Source: CAD feature listing. Evaluate the final solid. Frame: model axes, mm. Give positions to 0.01 mm unless a question says otherwise; leave off trailing zeros. Write each loop counter-clockwise with the first axis right and the second up, starting at its lowest first coordinate (ties: lowest second). Pieces come first, ordered by that corner, then holes. Notation, with made-up numbers: M -10.75,19 L -2.75,19 A22 cw -2.75,40 Z; hole C 44,39.25 d2. An arc over 180 degrees is marked long. Answer as a JSON object with one key per item and string values. Group by question number.
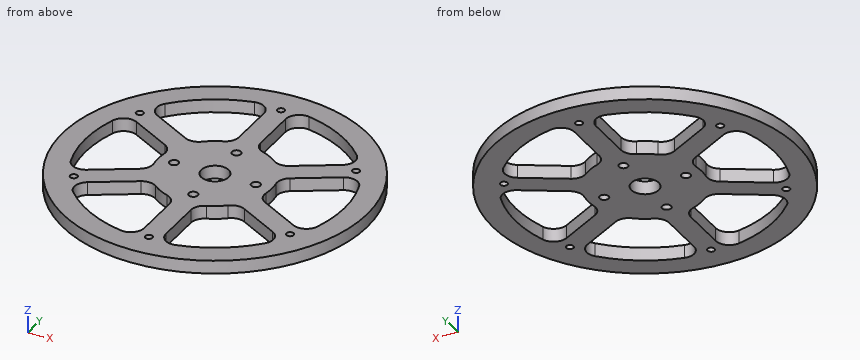
Autodesk Inventor part; units mm, degrees
ref_plane "YZ Plane" through (0, 0, 0) normal (1, 0, 0) x (0, 1, 0)
ref_plane "XZ Plane" through (0, 0, 0) normal (0, 1, 0) x (-1, 0, 0)
ref_plane "XY Plane" through (0, 0, 0) normal (0, 0, 1) x (1, 0, 0)
sketch "スケッチ1" plane through (0, 0, 0) normal (0, 0, 1) x (1, 0, 0)
  circle A0 centre (0, 0) radius 67
  circle A1 centre (0, 0) radius 57
  circle A2 centre (0, 0) radius 25
  line L0 (0, 0) -> (0, 67)
  circle A3 centre (0, 0) radius 6.05
  line L1 (4.7669, 0.7625) -> (4.7669, 66.8302)
  line L2 (4.7669, 0.7625) -> (70.8346, 0.7625) construction
  line L3 (-4.7669, 0.7625) -> (-4.7669, 66.8302)
  line L4 (-3.0438, -3.747) -> (-60.2601, 29.2869)
  line L5 (1.7231, 4.5095) -> (-55.4932, 37.5433)
  line L6 (1.7231, -4.5095) -> (-55.4932, -37.5433)
  line L7 (-3.0438, 3.747) -> (-60.2601, -29.2869)
  line L8 (4.7669, -0.7625) -> (4.7669, -66.8302)
  line L9 (-4.7669, -0.7625) -> (-4.7669, -66.8302)
  line L10 (3.0438, 3.747) -> (60.2601, -29.2869)
  line L11 (-1.7231, -4.5095) -> (55.4932, -37.5433)
  line L12 (-1.7231, 4.5095) -> (55.4932, 37.5433)
  line L13 (3.0438, -3.747) -> (60.2601, 29.2869)
  point P0 (4.7669, 56.8003)
  point P1 (46.8071, 32.5284)
  point P2 (18.87, 16.3989)
  point P3 (4.7669, 24.5413)
  point P4 (-4.7669, 56.8003)
  point P5 (-4.7669, 24.5413)
  point P6 (-18.87, 16.3989)
  point P7 (-46.8071, 32.5284)
  point P8 (51.574, -24.2719)
  point P9 (23.6368, -8.1424)
  point P10 (23.6368, 8.1424)
  point P11 (51.574, 24.2719)
  point P12 (4.7669, -56.8003)
  point P13 (4.7669, -24.5413)
  point P14 (18.87, -16.3989)
  point P15 (46.8071, -32.5284)
  point P16 (-46.8071, -32.5284)
  point P17 (-18.87, -16.3989)
  point P18 (-4.7669, -24.5413)
  point P19 (-4.7669, -56.8003)
  point P20 (-51.574, 24.2719)
  point P21 (-23.6368, 8.1424)
  point P22 (-23.6368, -8.1424)
  point P23 (-51.574, -24.2719)
  dimension "d0" = 134
  dimension "d1" = 114
  dimension "d2" = 50
  dimension "d3" = 12.1
  dimension "d4" = 90
  dimension "d7" = 360
extrude "押し出し1" add sketch "スケッチ1" along normal blind 5.8 contours A0 L10 A1 L13 | L13 A1 L12 A0 | A0 L11 A1 L10 | L12 A1 L1 A0 | L13 A2 L12 A1 | A0 L8 A1 L11 | A1 L11 A2 L10 | L1 A1 L0 A0 | L13 L10 A3 L1 L12 A2 | A2 L10 L13 | A0 L9 A1 L8 | A2 L11 L8 A3 L13 L10 | L0 A1 L3 A0 | L1 A2 L0 A1 | L12 L1 A2 | L13 A3 L10 | A0 L6 A1 L9 | A1 L9 A2 L8 | A2 L8 L11 | L3 A1 L5 A0 | L0 A2 L3 A1 | L1 L12 A3 L0 A2 | L1 A3 L12 | A0 L7 A1 L6 | A2 L9 L6 A3 L11 L8 | L11 A3 L8 | L5 A1 L4 A0 | L0 A3 L5 L3 A2 | A0 L4 A1 L7 | A1 L7 A2 L6 | A2 L6 L9 | L5 A2 L4 A1 | L3 L5 A2 | A2 L7 L4 A3 L9 L6 | L9 A3 L6 | L5 L3 A3 L7 L4 A2 | L5 A3 L3 | A2 L4 L7 | L7 A3 L4
sketch "スケッチ2" plane through (0, 0, 5.8) normal (0, 0, 1) x (1, 0, 0)
  point P0 (0, 0)
  point P1 (0, 18)
  point P2 (-18, 0)
  point P3 (0, -18)
  point P4 (18, 0)
  point P5 (0, 55)
  point P6 (-47.6314, 27.5)
  point P7 (-47.6314, -27.5)
  point P8 (0, -55)
  point P9 (47.6314, -27.5)
  point P10 (47.6314, 27.5)
  dimension "d11" = 18
  dimension "d14" = 360
  dimension "d16" = 55
  dimension "d19" = 360
hole "穴1" at (0, 18, 5.8) at (-18, 0, 5.8) at (0, -18, 5.8) at (18, 0, 5.8) direction (0, 0, -1) diameter 4 end through all
hole "穴2" at (0, 55, 5.8) at (-47.6314, 27.5, 5.8) at (-47.6314, -27.5, 5.8) at (0, -55, 5.8) at (47.6314, -27.5, 5.8) at (47.6314, 27.5, 5.8) direction (0, 0, -1) diameter 3.2 end through all
fillet "フィレット1" radius 6 24 edges at (-51.574, 24.2719, 2.9) (-51.574, -24.2719, 2.9) (-23.6368, -8.1424, 2.9) (-23.6368, 8.1424, 2.9) (-46.8071, 32.5284, 2.9) (-18.87, 16.3989, 2.9) (-4.7669, 24.5413, 2.9) (-4.7669, 56.8003, 2.9) (4.7669, 56.8003, 2.9) (4.7669, 24.5413, 2.9) (18.87, 16.3989, 2.9) (46.8071, 32.5284, 2.9) (51.574, 24.2719, 2.9) (23.6368, 8.1424, 2.9) (23.6368, -8.1424, 2.9) (51.574, -24.2719, 2.9) (46.8071, -32.5284, 2.9) (18.87, -16.3989, 2.9) (4.7669, -24.5413, 2.9) (4.7669, -56.8003, 2.9) (-4.7669, -56.8003, 2.9) (-4.7669, -24.5413, 2.9) (-18.87, -16.3989, 2.9) (-46.8071, -32.5284, 2.9)
properties part number "TH22_POM_roller_sn" material "ABS プラスチック"
(1) Section C-C, the plane x = -18. Return loops of the section in (y, z), plus the area to 3 significant figures.
(2) Section B-B, the plane x = 0. Return loops of the section in (y, z).
(3) Section D-D, the plane y = -40.5. Return loops of the section in (x, z), plus the area to 3 significant figures.
(4) Contact query for flat-ended pins moving along their axis: pin 1 Ø3 at (y, z) = (-43.5, 1.5) entering from -X; pin 2 Ø2 at (y, z) = (-37.5, 5) entering from +X; pin 3 Ø2 at (x, z) = (-29.5, 4) entering from -Y. Output: stop coordinate, or through.
(5) Ray query, L1, parallel to Y at x = 0, z = 2.4; L2, parallel to X at y = 50, z = 5.45; L3, parallel to X at y = -26.5, z = 2.6. Return the intervals inside material, ascending. Write a range as [from, to].
(6) Section A-A, the plane y = 0. Return loops of the section in (x, z), plus the area to 3 significant figures.
Reported:
{
 "1": {"outline": "M -64.54,0 L -54.08,0 L -54.08,5.8 L -64.54,5.8 Z; M -18.13,0 L -2,0 L -2,5.8 L -18.13,5.8 Z; M 2,0 L 18.13,0 L 18.13,5.8 L 2,5.8 Z; M 54.08,0 L 64.54,0 L 64.54,5.8 L 54.08,5.8 Z", "area": "308 mm2"},
 "2": {"outline": "M -67,0 L -56.6,0 L -56.6,5.8 L -67,5.8 Z; M -53.4,0 L -20,0 L -20,5.8 L -53.4,5.8 Z; M -16,0 L -6.05,0 L -6.05,5.8 L -16,5.8 Z; M 6.05,0 L 16,0 L 16,5.8 L 6.05,5.8 Z; M 20,0 L 53.4,0 L 53.4,5.8 L 20,5.8 Z; M 56.6,0 L 67,0 L 67,5.8 L 56.6,5.8 Z"},
 "3": {"outline": "M -53.37,0 L -40.11,0 L -40.11,5.8 L -53.37,5.8 Z; M -4.77,0 L 4.77,0 L 4.77,5.8 L -4.77,5.8 Z; M 40.11,0 L 53.37,0 L 53.37,5.8 L 40.11,5.8 Z", "area": "209 mm2"},
 "4": {"pin 1": "stops at x = -52.2", "pin 2": "stops at x = 56.18", "pin 3": "stops at y = -60.64"},
 "5": {"L1": "y = [-67, -56.6], [-53.4, -20], [-16, -6.05], [6.05, 16], [20, 53.4], [56.6, 67]", "L2": "x = [-44.6, -27.37], [-4.77, 4.77], [27.37, 44.6]", "L3": "x = [-61.54, -48.88], [-46.38, -36.37], [-5.35, 5.35], [36.37, 46.38], [48.88, 61.54]"},
 "6": {"outline": "M -67,0 L -57,0 L -57,5.8 L -67,5.8 Z; M -25,0 L -20,0 L -20,5.8 L -25,5.8 Z; M -16,0 L -6.05,0 L -6.05,5.8 L -16,5.8 Z; M 6.05,0 L 16,0 L 16,5.8 L 6.05,5.8 Z; M 20,0 L 25,0 L 25,5.8 L 20,5.8 Z; M 57,0 L 67,0 L 67,5.8 L 57,5.8 Z", "area": "289 mm2"}
}
